Geometry: final body of the model. Coordinates: model frame, mm. Face numbers are marked on the shaded views. A direction names the side the tool comes from. Round coordinates to 2 decimals unless told otherwise and drop trailing zeros. Loops run counter-clockwise (first coordinate to the right, second up) from the corner with the lowest first, then second, coordinate; pieces in that order, holes last. Notation, with made-up numbers: (-7, 35) - (9, 35) arc R26 cw to (9, 54) - close; hole circle Ø3 at (81.5, 9.25). An arc over 180 degrees is marked (long way). Answer as a JSON object with one key per item and string values. Group by question number.
Item 1: Section C-C (x = -64). Return the cut outline in (y, z).
Item 2: First-contact query: pin 1 (3 mm diameter, centred on x = -63.5, y = -11, fed in from -Z); pin 2 (2 mm diameter, centred on x = -8.5, z = -6.5, fed in from -Y); pin 3 (2 mm diameter, centred on x = -12, y = -8, fed in from +Z). Flat tips, straight axial feed; report the tip coordinate or a pass-through.
Item 3: Section B-B (z = 0). Return the cut outline in (x, y), plus the area to 3 significant figures.
Item 4: Section A-A (y = -7). Return the cut outline in (x, z).
Item 5: Reachability of the marked faces 1 and 2 from +Z, -Z, +X, -X, +Y, -Y: full face, straight path, thin tool, end or side. Return the list, or none.
Item 6: Line query: line 1 (X direction, y = -6, z = -8); line 2 (X direction, y = -11.5, z = 3.5); line 3 (Z direction, x = -55, y = -6.75). Output: solid intervals per line, ascending.
```python
from build123d import *

# Parameters (mm, degrees)
SKETCH2_R           = 5
BOSS_EXTRUDE1_DEPTH = 85


with BuildPart() as part:
    # Sketch1 → Revolve2 (revolve)
    with BuildSketch(Plane.XY):
        with BuildLine():
            ThreePointArc((6.40625, 0), (4.267173955, 2.473809592), (1.510462881, 0.714285714))
            ThreePointArc((1.510462881, 0.714285714), (1.149762338, 0.198216274), (0.552148034, 0))
            Line((0.552148034, 0), (-2.739648034, 0))
            ThreePointArc((-2.739648034, 0), (-3.337262338, 0.198216274), (-3.697962881, 0.714285714))
            ThreePointArc((-3.697962881, 0.714285714), (-6.454673955, 2.473809592), (-8.59375, 0))
            Line((-8.59375, 0), (-8.59375, -2))
            Line((-8.59375, -2), (6.40625, -2))
            Line((6.40625, -2), (6.40625, 0))
        make_face()
    revolve(axis=Axis((11.035645008, -7, 0), (-1, 0, 0)))

    # Sketch2 → Boss-Extrude1 (add)
    with BuildSketch(Plane(origin=(6.40625, 0, 0), x_dir=(0, 0, -1), z_dir=(1, 0, 0))):
        with Locations((0, -7)):
            Circle(SKETCH2_R)
    extrude(amount=-BOSS_EXTRUDE1_DEPTH)


solid = part.part
```
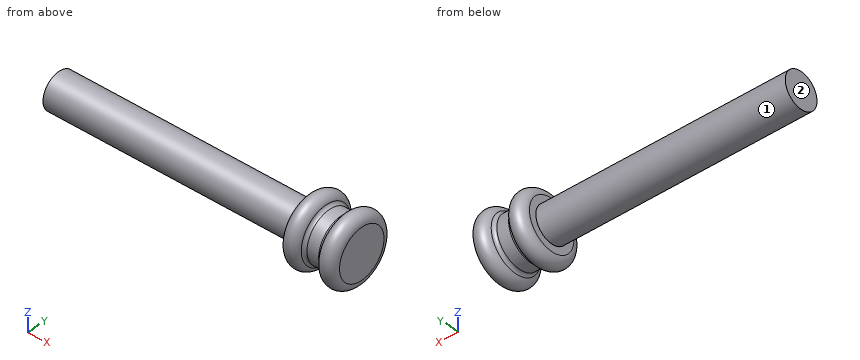
Values:
{
 "1": {"outline": "circle Ø10 at (-7, 0)"},
 "2": {"pin 1": "stops at z = -4.33", "pin 2": "stops at y = -13.68", "pin 3": "stops at z = 5"},
 "3": {"outline": "(-78.59, -12) - (-8.59, -12) - (-8.59, -14) arc R2.5 ccw to (-3.7, -14.71) arc R1 cw to (-2.74, -14) - (0.55, -14) arc R1 cw to (1.51, -14.71) arc R2.5 ccw to (6.41, -14) - (6.41, 0) arc R2.5 ccw to (1.51, 0.71) arc R1 cw to (0.55, 0) - (-2.74, 0) arc R1 cw to (-3.7, 0.71) arc R2.5 ccw to (-8.59, 0) - (-8.59, -2) - (-78.59, -2) - close", "area": "950 mm^2"},
 "4": {"outline": "(-78.59, -5) - (-8.59, -5) - (-8.59, -7) arc R2.5 ccw to (-3.7, -7.71) arc R1 cw to (-2.74, -7) - (0.55, -7) arc R1 cw to (1.51, -7.71) arc R2.5 ccw to (6.41, -7) - (6.41, 7) arc R2.5 ccw to (1.51, 7.71) arc R1 cw to (0.55, 7) - (-2.74, 7) arc R1 cw to (-3.7, 7.71) arc R2.5 ccw to (-8.59, 7) - (-8.59, 5) - (-78.59, 5) - close"},
 "5": {"face 1": "-X", "face 2": "+Z, -Z, -X, +Y, -Y"},
 "6": {"line 1": "x = -8.36 to -3.83, 1.64 to 6.17", "line 2": "x = -8.59 to 6.41", "line 3": "z = -4.99 to 4.99"}
}
